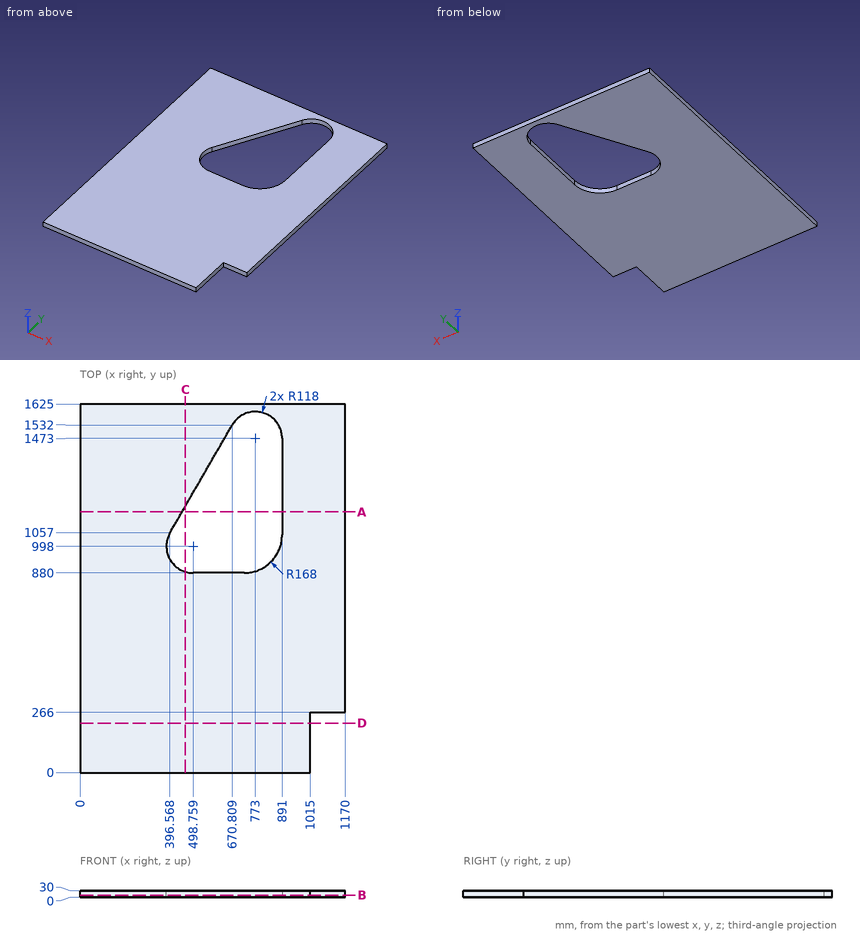
The drawing under review shows one solid part. Ordinate dimensions are in mm from its lowest x, y, z. Round coordinates to 2 decimals unless told otherwise and drop trailing zeros. Loops run counter-clockwise (first coordinate to the right, second up) from the corner with the lowest first, then second, coordinate; pieces in that order, holes last.
Item 1: Take a section at D-D (y = 218). Write out the cut boundary in (x, z).
Determined:
outline: (0, 0) - (1015, 0) - (1015, 30) - (0, 30) - close
Item 2: For line 1 (X direction, y = 1056.5, z = 12.5); line 2 (X direction, y = 129, z = 9.5); line 3 (Y direction, x = 734.5, z = 29) (1 decimal), list the stretches that pass through material, from the lowest coordinate up.
Determined:
line 1: x = 0 to 396.28, 891 to 1170
line 2: x = 0 to 1015
line 3: y = 0 to 880.4, 1584.5 to 1625
Item 3: Take a section at C-C (x = 464). Write out the cut boundary in (y, z) (1 decimal).
Determined:
outline: (0, 0) - (885.2, 0) - (885.2, 30) - (0, 30) - close; (1173.8, 0) - (1625, 0) - (1625, 30) - (1173.8, 30) - close
Item 4: Take a section at A-A (y = 1149). Write out the cut boundary in (x, z), then the cut area to 3 significant figures.
Determined:
outline: (0, 0) - (449.68, 0) - (449.68, 30) - (0, 30) - close; (891, 0) - (1170, 0) - (1170, 30) - (891, 30) - close
area: 21,900 mm2
Item 5: Take a section at B-B (z = 10). Write out the cut boundary in (x, y), then the cut area to 3 significant figures.
Determined:
outline: (0, 0) - (1015, 0) - (1015, 266) - (1170, 266) - (1170, 1625) - (0, 1625) - close; hole (396.57, 1057) arc R118 ccw to (498.76, 880) - (723, 880) arc R168 ccw to (891, 1048) - (891, 1473) arc R118 ccw to (670.81, 1532) - close
area: 1,600,000 mm2
